```python
from build123d import *

# Parameters (mm, degrees)
BASE_FLANGE1_DEPTH = 7.5
SKETCH6_R          = 1.25
CUT_EXTRUDE1_DEPTH = 10
CUT_EXTRUDE2_DEPTH = 10
FILLET1_R          = 1


# Sheet-metal steps are written as plain solids
with BuildPart() as part:
    # Base-Flange1: sheet metal written as solids
    # Sketch1 → Base-Flange1 (new, symmetric)
    with BuildSketch(Plane.XY):
        with BuildLine():
            Line((-17.75, 2.75), (-13.4866, 2.75))
            ThreePointArc((-13.4866, 2.75), (-12.965745145, 2.534254855), (-12.75, 2.0134))
            Line((-12.75, 2.0134), (-12.75, 1.2366))
            ThreePointArc((-12.75, 1.2366), (-12.387808246, 0.362191754), (-11.5134, 0))
            Line((-11.5134, 0), (11.5134, 0))
            ThreePointArc((11.5134, 0), (12.387808246, 0.362191754), (12.75, 1.2366))
            Line((12.75, 1.2366), (12.75, 2.0134))
            ThreePointArc((12.75, 2.0134), (12.965745145, 2.534254855), (13.4866, 2.75))
            Line((13.4866, 2.75), (17.75, 2.75))
            Line((17.75, 2.75), (17.75, 3.25))
            Line((17.75, 3.25), (13.4866, 3.25))
            ThreePointArc((13.4866, 3.25), (12.612191754, 2.887808246), (12.25, 2.0134))
            Line((12.25, 2.0134), (12.25, 1.2366))
            ThreePointArc((12.25, 1.2366), (12.034254855, 0.715745145), (11.5134, 0.5))
            Line((11.5134, 0.5), (-11.5134, 0.5))
            ThreePointArc((-11.5134, 0.5), (-12.034254855, 0.715745145), (-12.25, 1.2366))
            Line((-12.25, 1.2366), (-12.25, 2.0134))
            ThreePointArc((-12.25, 2.0134), (-12.612191754, 2.887808246), (-13.4866, 3.25))
            Line((-13.4866, 3.25), (-17.75, 3.25))
            Line((-17.75, 3.25), (-17.75, 2.75))
        make_face()
    extrude(amount=BASE_FLANGE1_DEPTH, both=True)

    # Sketch6 → Cut-Extrude1 (cut)
    with BuildSketch(Plane.XZ.offset(-2.75)):
        with Locations(Location((-15, -0.75, 0), (0, 0, 270))):
            Circle(SKETCH6_R)
        with Locations(Location((15, -0.75, 0), (0, 0, 270))):
            Circle(SKETCH6_R)
    extrude(amount=-CUT_EXTRUDE1_DEPTH, mode=Mode.SUBTRACT)

    # Sketch7 → Cut-Extrude2 (cut)
    with BuildSketch(Plane.XZ):
        with BuildLine():
            ThreePointArc((-6.470027047, 5.279972953), (-4.843681451, 5.279972953), (-4.843681451, 6.906318549))
            ThreePointArc((-4.843681451, 6.906318549), (0, 18.599999999), (4.843681451, 6.906318549))
            ThreePointArc((4.843681451, 6.906318549), (4.843681451, 5.279972953), (6.470027047, 5.279972953))
            ThreePointArc((6.470027047, 5.279972953), (0, 20.899999999), (-6.470027047, 5.279972953))
        make_face()
    extrude(amount=-CUT_EXTRUDE2_DEPTH, mode=Mode.SUBTRACT)

    # Fillet1
    fillet1_edges = [part.edges().sort_by_distance(p)[0] for p in [
        (8.103085831, 0.25, 7.5),
        (-8.103085831, 0.25, 7.5),
        (-5.372150407, 0.25, 7.5),
        (5.372150407, 0.25, 7.5),
    ]]
    fillet(fillet1_edges, radius=FILLET1_R)


solid = part.part
```
Input: part model. Units: mm. Frame: model coordinates. A direction names the side the tool comes from. Round coordinates to 2 decimals unless told otherwise and drop trailing zeros. Write each loop counter-clockwise with the first axis right and the second up, starting at its lowest first coordinate (ties: lowest second). Pieces come first, ordered by that corner, then holes. Notation, with made-up numbers: (20.5, -37.5) - (28.5, -37.5) arc R22 ccw to (28.5, -20.5) - close; hole circle Ø11 at (-27.75, -15). An arc over 180 degrees is marked (long way). Write item = value, one per line.
(1) Section query B-B on z = -1.5. Output: boundary loops of the cut face in (x, y), then the cut area to 3 significant figures.
Geometry check:
outline = (-17.75, 2.75) - (-16, 2.75) - (-16, 3.25) - (-17.75, 3.25) - close; (-14, 2.75) - (-13.49, 2.75) arc R0.74 cw to (-12.75, 2.01) - (-12.75, 1.24) arc R1.24 ccw to (-11.51, 0) - (11.51, 0) arc R1.24 ccw to (12.75, 1.24) - (12.75, 2.01) arc R0.74 cw to (13.49, 2.75) - (14, 2.75) - (14, 3.25) - (13.49, 3.25) arc R1.24 ccw to (12.25, 2.01) - (12.25, 1.24) arc R0.74 cw to (11.51, 0.5) - (-11.51, 0.5) arc R0.74 cw to (-12.25, 1.24) - (-12.25, 2.01) arc R1.24 ccw to (-13.49, 3.25) - (-14, 3.25) - close; (16, 2.75) - (17.75, 2.75) - (17.75, 3.25) - (16, 3.25) - close
area = 17.7 mm^2
(2) Section query C-C on y = 0.9. Output: boundary loops of the cut face in (x, z), then the cut area to 3 significant figures.
Geometry check:
outline = (-12.7, -7.5) - (-12.17, -7.5) - (-12.17, 7.5) - (-12.7, 7.5) - close; (12.17, -7.5) - (12.7, -7.5) - (12.7, 7.5) - (12.17, 7.5) - close
area = 16.0 mm^2
(3) Material intervals for probe 1 along X at (y, z) = (1.15, 4.75); probe 2 along X at (y, z) = (3.05, -0.75); probe 3 along X at (y, z) = (3, -0.75), sorted ascending.
Geometry check:
probe_1 = -12.75 to -12.24, 12.24 to 12.75
probe_2 = -17.75 to -16.25, -13.75 to -12.81, 12.81 to 13.75, 16.25 to 17.75
probe_3 = -17.75 to -16.25, -13.75 to -12.74, 12.74 to 13.75, 16.25 to 17.75
(4) Pull-direction query (X, two-part tool) for faces 4 (the cylindrical face through (12.378, 0.353, 0.105)), 5 (the flat face through (16.12, 3.25, 0.11)), 6 (the cylindrical face through (5.1, 0.246, 5.087)); classes: +X half, -X half, draft (parallel to the pull), parting line (faces both ways), or undercut.
Geometry check:
face_4 = +X half
face_5 = draft
face_6 = undercut
(5) Section query D-D on x = -10. Output: boundary loops of the cut face in (y, z).
Geometry check:
outline = (0, -7.5) - (0.5, -7.5) - (0.5, 7.5) - (0, 7.5) - close
(6) Access query for faces 1 (the cylindrical face through (12.622, 2.897, 0.105)), 2 (the cylindrical face through (-7.213, 0.246, 6.12)), 3 (the flat face through (17, 2.75, 0)). Directions: +Z, -Z, +X, -X, +Y, -Y. A direction counts if a zero-diameter tool reaches every point of the face in a straight line with its end or side. Return the directions, or none.
Geometry check:
face_1 = +Z, -Z, +Y
face_2 = +Z, +Y, -Y
face_3 = +Z, -Z, +X, -Y
(7) Section query A-A on x = -15. Output: boundary loops of the cut face in (y, z), then the cut area to 3 significant figures.
Geometry check:
outline = (2.75, -7.5) - (3.25, -7.5) - (3.25, -2) - (2.75, -2) - close; (2.75, 0.5) - (3.25, 0.5) - (3.25, 7.5) - (2.75, 7.5) - close
area = 6.25 mm^2
(8) Contact query for flat-ended pins moving along their axis: pin 1 Ø2 at (x, z) = (-14.5, 3.5) entering from -Y; pin 2 Ø0.6 at (y, z) = (1.5, -3.5) entering from -X; pin 3 Ø0.6 at (y, z) = (1.5, 3) entering from +X. Output: stop coordinate, or through.
Geometry check:
pin_1 = 2.75
pin_2 = -12.75
pin_3 = 12.75
